Verification items for the finished model (mm, model axes). Face numbers are marked on the shaded views. Round coordinates to 2 decimals unless told otherwise and drop trailing zeros. Order: outer loops, then holes, each group sorted by start corner. A loop starts at its lowest first (then second) coordinate and runs counter-clockwise, first axis right, second up. Notation, with made-up numbers: (76.25, -3.5) -> (92.25, -3.5) arc R21 cw to (92.25, 0.5) -> close; hole circle Ø6 at (55.25, 43). An arc over 180 degrees is marked (long way). Put each result on its own line as item: value.
```python
from build123d import *

# Parameters (mm, degrees)
SKETCH1_R           = 12.7
SKETCH1_R_2         = 8.73125
BOSS_EXTRUDE1_DEPTH = 6.35
SKETCH2_R           = 12.7
SKETCH2_R_2         = 7.9375
BOSS_EXTRUDE2_DEPTH = 23.8125
SKETCH5_R           = 12.7
BOSS_EXTRUDE4_DEPTH = 65.0875
SKETCH6_R           = 6.35
SKETCH3_R           = 4.7625


with BuildPart() as part:
    # Sketch1 → Boss-Extrude1 (new body)
    with BuildSketch(Plane.XY):
        Circle(SKETCH1_R)
        Circle(SKETCH1_R_2, mode=Mode.SUBTRACT)
    extrude(amount=BOSS_EXTRUDE1_DEPTH)



with BuildPart() as body_2:
    # Sketch2 → Boss-Extrude2 (new body)
    with BuildSketch(Plane.XY.offset(71.4375)):
        Circle(SKETCH2_R)
        Circle(SKETCH2_R_2, mode=Mode.SUBTRACT)
    extrude(amount=BOSS_EXTRUDE2_DEPTH)


with BuildPart() as part_1:
    add(part.part)

    add(body_2.part)  # Boss-Extrude4 merges body 2
    # Sketch5 → Boss-Extrude4 (add)
    with BuildSketch(Plane.XY.offset(6.35)):
        Circle(SKETCH5_R)
    extrude(amount=BOSS_EXTRUDE4_DEPTH)

    # Sketch6 → Cut-Loft1 section 0
    with BuildSketch(Plane.XY.offset(6.35)):
        Circle(SKETCH6_R)
    # Sketch3 → Cut-Loft1 section 1
    with BuildSketch(Plane(origin=(0, 0, 71.4375), x_dir=(-1, 0, 0), z_dir=(0, 0, -1))):
        Circle(SKETCH3_R)
    loft(mode=Mode.SUBTRACT)


solid = part_1.part
```
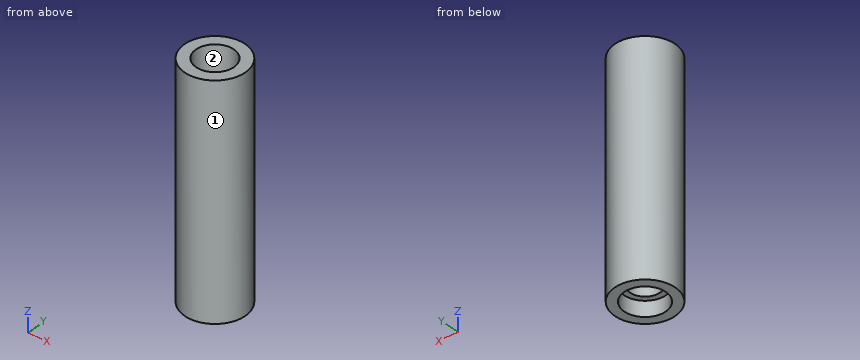
Item 1: Sectioned sample at A-A, the plane x = 0. Record the boundary of the cut face in (y, z).
Geometry check:
outline: (-12.7, 0) -> (-8.73, 0) -> (-8.73, 6.35) -> (-6.35, 6.35) -> (-4.76, 71.44) -> (-7.94, 71.44) -> (-7.94, 95.25) -> (-12.7, 95.25) -> close; (4.76, 71.44) -> (6.35, 6.35) -> (8.73, 6.35) -> (8.73, 0) -> (12.7, 0) -> (12.7, 95.25) -> (7.94, 95.25) -> (7.94, 71.44) -> close
Item 2: Sectioned sample at D-D, the plane z = 48.5. Record the boundary of the cut face in (x, y).
Geometry check:
outline: circle Ø25.4 at (0, 0); hole circle Ø10.64 at (0, 0)
Item 3: Material ranges on line 1 along Y through (x, z) = (0, 73.5); line 2 along X through (y, z) = (0.25, 80); line 3 along Y through (x, z) = (0, 2.75), recorded low to high.
Geometry check:
line 1: -12.7 to -7.94, 7.94 to 12.7
line 2: -12.7 to -7.93, 7.93 to 12.7
line 3: -12.7 to -8.73, 8.73 to 12.7
Item 4: Sectioned sample at B-B, the plane z = 11. Record the boundary of the cut face in (x, y), then the cut area to 3 significant figures.
Geometry check:
outline: circle Ø25.4 at (0, 0); hole circle Ø12.47 at (0, 0)
area: 385 mm2
Item 5: Sectioned sample at C-C, the plane x = -10. Record the boundary of the cut face in (y, z), then the cut area to 3 significant figures.
Geometry check:
outline: (-7.83, 0) -> (7.83, 0) -> (7.83, 95.25) -> (-7.83, 95.25) -> close
area: 1,490 mm2
Item 6: Release check for a two-part mould opening along Y. For the marked faces 1 and 2 record: pulls with the +Y half, pulls with the -Y half, needs draft (parallel to the pull), parting line crosses it, or undercut.
Geometry check:
face 1: parting line crosses it
face 2: undercut
Item 7: Depth check by flat-ended pin: pin 1 Ø14 at (x, y) = (0, 0) entering from +Z; pin 2 Ø1 at (y, z) = (-6.5, 37) entering from -X; pin 3 Ø5 at (y, z) = (7, 33) entering from +X. Enter the tip coordinate at first touch or a pass-through.
Geometry check:
pin 1: z = 71.44
pin 2: x = -11.19
pin 3: x = 11.88
